```python
from build123d import *

# Parameters (mm, degrees)
F0_W      = 73.025
F0_H      = 101.6
F1_DEPTH  = 508
F2_R      = 7.62
F3_DEPTH  = 101.601
F4_R      = 7.62
F5_DEPTH  = 1430.3385
F8_DEPTH  = 1498.6
F10_DEPTH = 76.2


with BuildPart() as f1:
    # F0 (on Front) → F1 (new body)
    with BuildSketch(Plane.XZ):
        with Locations((-678.65625, 50.8)):
            Rectangle(F0_W, F0_H)
    extrude(amount=-F1_DEPTH)


with BuildPart() as f1b:
    # F0 (on Front) → F1, piece 2 (new body)
    with BuildSketch(Plane.XZ):
        with Locations((678.65625, 50.8)):
            Rectangle(F0_W, F0_H)
    extrude(amount=-F1_DEPTH)


with BuildPart() as f3_tool:
    # F2 (on face) → F3 (new body, through all)
    with BuildSketch(Plane(origin=(0, 0, 0), x_dir=(1, 0, 0), z_dir=(0, 0, -1))):
        with Locations((-678.65625, -25.4)):
            Circle(F2_R)
        with Locations((-678.65625, -114.3)):
            Circle(F2_R)
        with Locations((-678.65625, -203.2)):
            Circle(F2_R)
        with Locations((678.65625, -25.4)):
            Circle(F2_R)
        with Locations((678.65625, -114.3)):
            Circle(F2_R)
        with Locations((678.65625, -203.2)):
            Circle(F2_R)
    extrude(amount=-F3_DEPTH)


with BuildPart() as f1_1:
    add(f1.part)

    # F3: cut by f3_tool
    add(f3_tool.part, mode=Mode.SUBTRACT)


with BuildPart() as f1b_1:
    add(f1b.part)

    # F3: cut by f3_tool
    add(f3_tool.part, mode=Mode.SUBTRACT)


with BuildPart() as f5_tool:
    # F4 (on face) → F5 (new body, through all)
    with BuildSketch(Plane(origin=(-715.16875, 0, 0), x_dir=(0, -1, 0), z_dir=(-1, 0, 0))):
        with Locations((-114.3, 63.5)):
            Circle(F4_R)
        with Locations((-55.88, 35.56)):
            Circle(F4_R)
        with Locations((-35.56, 63.5)):
            Circle(F4_R)
    extrude(amount=-F5_DEPTH)


with BuildPart() as f1_2:
    add(f1_1.part)

    # F5: cut by f5_tool
    add(f5_tool.part, mode=Mode.SUBTRACT)



with BuildPart() as f1b_2:
    add(f1b_1.part)

    # F5: cut by f5_tool
    add(f5_tool.part, mode=Mode.SUBTRACT)


with BuildPart() as f1_3:
    add(f1_2.part)

    add(f1b_2.part)  # F8 merges F1b
    # F7 (on offset) → F8 (join)
    with BuildSketch(Plane.YZ.offset(749.3)):
        Polygon((-38.1, 107.95), (0, 107.95), (0, 101.6), (229.8964709044, 101.6), (229.8964709044, 654.05), (-114.3, 654.05), (-114.3, 146.05), (-38.1, 146.05), align=None)
    extrude(amount=-F8_DEPTH)

    # F9 (on face) → F10 (join)
    with BuildSketch(Plane.YZ.offset(749.3)):
        Polygon((-114.3, 506.1743855476), (-111.125, 146.05), (-38.1, 146.05), (-38.1, 107.95), (0, 107.95), (0, 101.6), (210.1973444223, 101.6), (210.1973444223, 506.1743855476), align=None)
        with BuildLine():
            Line((-38.1, 146.05), (-111.125, 146.05))
            add(Edge.make_bspline(
                [(-111.125, 146.05), (-110.1389825344, 127.9860138893), (-100.2988577604, 117.881006452), (-101.5214413042, -130.5658881024), (101.1466756463, -23.6625690013), (210.1973444223, -22.5266236812)],
                knots=[0, 0, 0, 0, 0.1758084358, 0.5312599023, 1, 1, 1, 1], degree=3))
            Line((210.1973444223, -22.5266236812), (210.1973444223, 101.6))
            Line((210.1973444223, 101.6), (0, 101.6))
            Line((0, 101.6), (0, 107.95))
            Line((0, 107.95), (-38.1, 107.95))
            Line((-38.1, 107.95), (-38.1, 146.05))
        make_face()
    extrude(amount=F10_DEPTH)

    # F11: F1 across plane


with BuildPart() as f1_4:
    add(f1_3.part)
    add(f1_3.part.mirror(Plane.YZ))


solid = f1_4.part
```
The model under review builds one solid part; all positions refer to its coordinate system, in mm. A direction names the side the tool comes from. Round coordinates to 2 decimals unless told otherwise and drop trailing zeros. Write each loop counter-clockwise with the first axis right and the second up, starting at its lowest first coordinate (ties: lowest second). Pieces come first, ordered by that corner, then holes. Notation, with made-up numbers: (-8.5, 12.5) -> (26.5, 12.5) arc R14 ccw to (26.5, 30.5) -> close; hole circle Ø10 at (-39.75, 33). An arc over 180 degrees is marked (long way). Use CSV: the item, a comma, the result in double quotes.
Q1. Consider section D-D (z = 206). Give the boundary of the cut face in (x, y).
Checks:
outline,"(-825.5, -111.65) -> (-749.3, -111.65) -> (-749.3, -114.3) -> (749.3, -114.3) -> (749.3, -111.65) -> (825.5, -111.65) -> (825.5, 210.2) -> (749.3, 210.2) -> (749.3, 229.9) -> (-749.3, 229.9) -> (-749.3, 210.2) -> (-825.5, 210.2) -> close"
Q2. For faces 4 (the flat face through (10, -19, 107.95)), 5 (the flat face through (-679, 250, 0)), 6 (the flat face through (-679, 367, 101.6)), list the 3-axis set-ups (+Z, -Z, +X, -X, +Y, -Y) from which the entire face can be reached by the end or side of a thin tool; tool diameter is ignored.
Checks:
face 4,"-Z, -Y"
face 5,"-Z, +Y, -Y"
face 6,"+Z, +X, -X, +Y"
Q3. Consider section C-C (z = 466). Give the boundary of the cut face in (x, y).
Checks:
outline,"(-825.5, -113.95) -> (-749.3, -113.95) -> (-749.3, -114.3) -> (749.3, -114.3) -> (749.3, -113.95) -> (825.5, -113.95) -> (825.5, 210.2) -> (749.3, 210.2) -> (749.3, 229.9) -> (-749.3, 229.9) -> (-749.3, 210.2) -> (-825.5, 210.2) -> close"
Q4. Consider section B-B (x = 360). Give the boundary of the cut face in (y, z).
Checks:
outline,"(-114.3, 146.05) -> (-38.1, 146.05) -> (-38.1, 107.95) -> (0, 107.95) -> (0, 101.6) -> (229.9, 101.6) -> (229.9, 654.05) -> (-114.3, 654.05) -> close"
Q5. Consider section A-A (y = 350). Give the boundary of the cut face in (x, z).
Checks:
outline,"(-715.17, 0) -> (-642.14, 0) -> (-642.14, 101.6) -> (-715.17, 101.6) -> close; (642.14, 0) -> (715.17, 0) -> (715.17, 101.6) -> (642.14, 101.6) -> close"
Q6. To check wall thickness, follow probe 1 along X at (y, z) = (25, 33); probe 2 along X at (y, z) = (153.5, 3); probe 3 along Z at (x, y) = (-696, 114). State the ranges of each line that lie inside material, in increasing order. Write a range as [from, to].
Checks:
probe 1,"[-825.5, -749.3], [-715.17, -686.27], [-671.05, -642.14], [642.14, 671.05], [686.27, 715.17], [749.3, 825.5]"
probe 2,"[-825.5, -749.3], [-715.17, -642.14], [642.14, 715.17], [749.3, 825.5]"
probe 3,"[0, 55.89], [71.11, 654.05]"
Q7. For pin 1 Ø10 at (x, y) = (738.5, 158) entering from -Z; pin 2 Ø4 at (x, z) = (413, 435) entering from +Y; pin 3 Ø7.5 at (x, y) = (-675, 118) entering from -Z, all flat-tipped, find the tip position at first contact; note any pin that passes through.
Checks:
pin 1,"z = 101.6"
pin 2,"y = 229.9"
pin 3,"z = 0"
Q8. Mouldability with a two-part tool opening along X and no side actions: class faces 1 (the flat face through (787, 50, 506.174)), 2 (the flat face through (-732, 113, 101.6)), 3 (the flat face through (825.5, 46, 263)) as released by +X, released by -X, zero draft, split by the parting line, or undercut.
Checks:
face 1,"zero draft"
face 2,"undercut"
face 3,"released by +X"
